Source: CAD feature listing. Evaluate the final solid. Frame: model axes, mm. A direction names the side the tool comes from. Give positions to 0.01 mm unless a question says otherwise; leave off trailing zeros. Order: outer loops, then holes, each group sorted by start corner. A loop starts at its lowest first (then second) coordinate and runs counter-clockwise, first axis right, second up. Notation, with made-up numbers: M -31.75,-40 L -24.75,-40 A22 cw -24.75,-23 Z; hole C -24.75,-3 d9. An arc over 180 degrees is marked long. Return JSON: item names as keys, results as strings.
Autodesk Inventor part; units mm, degrees
ref_plane "YZ Plane" through (0, 0, 0) normal (1, 0, 0) x (0, 1, 0)
ref_plane "XZ Plane" through (0, 0, 0) normal (0, 1, 0) x (-1, 0, 0)
ref_plane "XY Plane" through (0, 0, 0) normal (0, 0, 1) x (1, 0, 0)
sketch "Sketch1" plane through (0, 0, 0) normal (0, 1, 0) x (-1, 0, 0)
  circle A0 centre (0, 0) radius 11.8999
  dimension "d0" = 23.7998
extrude "Extrusion1" add sketch "Sketch1" along normal blind 6.35
hole "Hole1" at (0, 0, 0) direction (0, 1, 0) diameter 6.7564 end through all counterbore diameter 11.1252 counterbore depth 1.5875
fillet "Fillet1" radius 3.175 1 edges at (11.8999, 0, 0)
properties part number "RoundRetainingClip"
1. Set-up query: faces 4 (the face through (2.056, 4.002, 2.681)), 5 (the face through (-1.671, 0.805, -5.306)). Return all of +Z, -Z, +X, -X, +Y, -Y with unobstructed straight access to the full face (end or side cutting, diameter ignored); none if empty.
Evaluation:
{"face 4": "+Y, -Y", "face 5": "-Y"}
2. Draft query along Z for faces 1 (the face through (0, 1.588, -4)), 2 (the face through (0, 0, -6)), 3 (the face through (9.443, 4.74, 7.241)). Return one class per face: pulls with the +Z half, pulls with the -Z half, needs draft (parallel to the pull), parting line crosses it, or undercut.
Evaluation:
{"face 1": "undercut", "face 2": "needs draft", "face 3": "parting line crosses it"}
3. Ray query, probe 1 along Z at (x, y) = (0, 4.9); probe 2 along Y at (x, z) = (-2.5, -3.5); probe 3 along Z at (x, y) = (0, 1.25). Return the intervals inside material, ascending.
Evaluation:
{"probe 1": "z = -11.9 to -3.38, 3.38 to 11.9", "probe 2": "y = 1.59 to 6.35", "probe 3": "z = -11.25 to -5.56, 5.56 to 11.25"}
4. First-contact query: pin 1 (2 mm diameter, centred on x = 3.5, y = 5.5, fed in from +Z); pin 2 (4 mm diameter, centred on x = 0, z = 0, fed in from -Y); pin 3 (1.5 mm diameter, centred on y = 1, z = 2.5, fed in from -X); pin 4 (2 mm diameter, centred on y = 5, z = -4, fed in from +X). Flat tips, straight axial feed; report the tip coordinate or a pass-through.
Evaluation:
{"pin 1": "stops at z = 11.63", "pin 2": "passes through", "pin 3": "stops at x = -11.32", "pin 4": "stops at x = 11.52"}
5. Section query D-D (y = 2.5). Return loops of the section in (x, z), then the cut area to 3 significant figures.
Evaluation:
{"outline": "C 0,0 d23.65; hole C 0,0 d6.76", "area": "404 mm^2"}
6. Section query C-C (y = 4.25). Return loops of the section in (x, z).
Evaluation:
{"outline": "C 0,0 d23.8; hole C 0,0 d6.76"}
